Check sheet for the modelled part. Datum: model origin and axes. Units: mm. A direction names the side the tool comes from. Round coordinates to 2 decimals unless told otherwise and drop trailing zeros. Loops run counter-clockwise (first coordinate to the right, second up) from the corner with the lowest first, then second, coordinate; pieces in that order, holes last. Notation, with made-up numbers: (76.25, 51) - (135.25, 51) arc R33 ccw to (135.25, 88) - close; hole circle Ø10 at (15, 34). An arc over 180 degrees is marked (long way). Answer in a Markdown table with one row per item. Add a question column.
(1) Cross-section at B-B on z = 0. Enter the section's corners in (x, y), then the cut area to 3 significant figures.
(2) Access from +Z, -Z, +X, -X, +Y, -Y to the whole of each face (thin tool, end or side, straight path). Record for faces 1 (the cylindrical face through (-0.9, -7.23, 2.86)), 2 (the flat face through (0, 15.308, 0)).
(3) Cross-section at D-D on z = 5.5. Enter the section's corners in (x, y), then the cut area to 3 significant figures.
(4) Thickness scan on line 1 along Y through (x, z) = (6, 2.25); line 2 along Y through (x, z) = (2, -3.5); line 3 along X through (y, z) = (1.25, -0.5). Record the ranges inside material, lowest first.
(5) Cross-section at C-C on y = -0.5. Enter the section's corners in (x, z), then the cut area to 3 significant figures.
(6) Mould release check, pull along Y, two halves, no side actions. Record for faces 3 (the cylindrical face through (-0.9, 4.45, 2.86)), 4 (the flat face through (0, -9.692, 0)), 5 (the flat face through (-2.24, -3.192, 2.24)), 6 (the cylindrical face through (9.274, -3.953, -2.059)): +Y half, -Y half, draft (parallel to the pull), parting line (faces both ways), or undercut.
(7) Cross-section at A-A on x = 0. Enter the section's corners in (y, z), then the cut area to 3 significant figures.
(8) Gauge pin test, flat ends, axial feed: pin 1 (8 mm diameter, centred on y = -1.5, z = -5, fed in from -X); pin 2 (1.5 mm diameter, centred on x = -7, z = 5, fed in from +Y); pin 3 (2 mm diameter, centred on x = 0.5, y = 4.5, fed in from -Z). Record the tip position at first contact, or that the pin passes through.
from build123d import *


with BuildPart() as part:
    # Эскиз1 → Повернуть2 (revolve)
    with BuildSketch(Plane.XY, mode=Mode.PRIVATE) as revolve_2_sk:
        with BuildLine():
            Line((3, 12.30781391), (3, -3.19218609))
            Line((3, -3.19218609), (9.5, -3.19218609))
            Line((9.5, -3.19218609), (9.5, -4.69218609))
            Line((9.5, -4.69218609), (3, -4.69218609))
            Line((3, -4.69218609), (3, -9.69218609))
            Line((3, -9.69218609), (0, -9.69218609))
            Line((0, -9.69218609), (0, 15.30781391))
            Line((0, 15.30781391), (3.25, 15.30781391))
            ThreePointArc((3.25, 15.30781391), (4.75, 13.80781391), (3.25, 12.30781391))
            Line((3.25, 12.30781391), (3, 12.30781391))
        make_face()
    revolve(revolve_2_sk.sketch.rotate(Axis((0, 15.673981191, 0), (0, -1, 0)), 90), axis=Axis((0, 15.673981191, 0), (0, -1, 0)))


solid = part.part
Answers:
| question | item | result |
|---|---|---|
| 1 | outline | (-9.5, -4.69) - (-3, -4.69) - (-3, -9.69) - (3, -9.69) - (3, -4.69) - (9.5, -4.69) - (9.5, -3.19) - (3, -3.19) - (3, 12.31) - (3.25, 12.31) arc R1.5 ccw to (3.25, 15.31) - (-3.25, 15.31) arc R1.5 ccw to (-3.25, 12.31) - (-3, 12.31) - (-3, -3.19) - (-9.5, -3.19) - close |
| 1 | area | 178 mm^2 |
| 2 | face 1 | -Y |
| 2 | face 2 | +Z, -Z, +X, -X, +Y |
| 3 | outline | (-7.75, -4.69) - (7.75, -4.69) - (7.75, -3.19) - (-7.75, -3.19) - close |
| 3 | area | 23.2 mm^2 |
| 4 | line 1 | y = -4.69 to -3.19 |
| 4 | line 2 | y = -4.69 to -3.19, 12.53 to 15.09 |
| 4 | line 3 | x = -2.96 to 2.96 |
| 5 | outline | circle Ø6 at (0, 0) |
| 5 | area | 28.3 mm^2 |
| 6 | face 3 | undercut |
| 6 | face 4 | -Y half |
| 6 | face 5 | undercut |
| 6 | face 6 | draft |
| 7 | outline | (-9.69, -3) - (-4.69, -3) - (-4.69, -9.5) - (-3.19, -9.5) - (-3.19, -3) - (12.31, -3) - (12.31, -3.25) arc R1.5 ccw to (15.31, -3.25) - (15.31, 3.25) arc R1.5 ccw to (12.31, 3.25) - (12.31, 3) - (-3.19, 3) - (-3.19, 9.5) - (-4.69, 9.5) - (-4.69, 3) - (-9.69, 3) - close |
| 7 | area | 178 mm^2 |
| 8 | pin 1 | stops at x = -9.4 |
| 8 | pin 2 | stops at y = -3.19 |
| 8 | pin 3 | stops at z = -3 |
